The model under review builds one solid part; all positions refer to its coordinate system, in mm. A direction names the side the tool comes from. Coordinates: 2 decimals unless noted, no trailing zeros. Loops run counter-clockwise (first coordinate to the right, second up) from the corner with the lowest first, then second, coordinate; pieces in that order, holes last. Notation, with made-up numbers: (-36, -11) - (20, -11) arc R19 ccw to (20, -7) - close; hole circle Ø2 at (38.5, 74). An arc over 180 degrees is marked (long way). One line per item, written item: value. Start each with the question number.
1. Insertion check: P1, Ø1.5, axis at y = 1.5, z = -10, coming from the +X side; P2, Ø1.5, axis at x = 34, y = 2, coming from the -Z side; P3, Ø1.5, axis at x = 7.5, y = 1, coming from the -Z side. Each pin has a flat end and moves straight along its axis. Give the tip position at first contact, or say it passes through.
2. Mouldability with a two-part tool opening along X and no side actions: class faces 1 (the face through (-52.23, 1.99, -52.13)), 2 (the face through (-1, 3, -15)), 3 (the face through (-13.922, 1.479, -11.116)), 4 (the face through (81.49, 1.52, 38.52)) as +X half, -X half, draft (parallel to the pull), parting line (faces both ways), or undercut.
3. We need section B-B, the plane z = 0. Give the boundary of the cut face in (x, y).
4. We need section D-D, the plane x = -34.5. Count the separate pieces of the cut face and the enclosed holes in it, then the cut area to 3 significant figures.
5. We need section C-C, the plane x = 0. Give the boundary of the cut face in (y, z), then the cut area to 3 significant figures.
6. To check wall thickness, follow line 1 (Z direction, x = -38.5, y = -6.75); line 2 (X direction, y = -3, z = 39.5); line 3 (Z direction, x = -39.1, y = 2.2). State the ranges of each line that lie inside material, in increasing order.
7. For faces 5 (the face through (-52.13, 1.99, 52.23)), 6 (the face through (-18.5, -8, -37.5)), 7 (the face through (-51.465, -3.944, -58.494)), list the 3-axis set-ups (+Z, -Z, +X, -X, +Y, -Y) from which the entire face can be reached by the end or side of a thin tool; tool diameter is ignored.
8. We need section A-A, the plane y = -2.75. Give the boundary of the cut face in (x, z), then the cut area to 3 significant figures.
from build123d import *

# Parameters (mm, degrees)
SKETCH1_W             = 120.2
SKETCH1_H             = 120.2
SKETCH1_W_2           = 110.2
SKETCH1_H_2           = 110.2
BOSS_EXTRUDE1_DEPTH   = 3
SKETCH3_W             = 25
SKETCH3_H             = 25
SKETCH3_R             = 3
SKETCH3_W_2           = 24.35
SKETCH3_H_2           = 24.35
BOSS_EXTRUDE3_DEPTH   = 3
FILLET1_R             = 12
SKETCH4_R             = 26.20371479
SKETCH4_R_2           = 18.5
BOSS_EXTRUDE4_DEPTH   = 3
SKETCH5_R             = 23
SKETCH5_R_2           = 20.5
BOSS_EXTRUDE5_DEPTH   = 8
SKETCH6_R             = 14.298791064
BOSS_EXTRUDE6_DEPTH   = 5.7
CIRPATTERN1_COUNT     = 4
SKETCH7_R             = 21.686675293
CUT_EXTRUDE1_DEPTH    = 5.7
SKETCH8_W             = 5.547879072
SKETCH8_H             = 55.825533157
SKETCH8_W_2           = 52.326060464
SKETCH8_H_2           = 5.547879072
BOSS_EXTRUDE7_DEPTH   = 3
BOSS_EXTRUDE8_DEPTH   = 3
BOSS_EXTRUDE9_DEPTH   = 3
CUT_EXTRUDE2_START    = -9
SKETCH12_R            = 20.5
CUT_EXTRUDE2_DEPTH    = 9
SKETCH14_R            = 1.812502671
CUT_EXTRUDE3_DEPTH    = 9
CIRPATTERN2_OUTLINE_R = 20.5
CIRPATTERN2_DEPTH     = 1


# Read off the part's stored shape, not the designer's step: CirPattern2
with BuildPart() as part:
    # Sketch1 → Boss-Extrude1 (new body)
    with BuildSketch(Plane(origin=(0, 0, 0), x_dir=(1, 0, 0), z_dir=(0, 1, 0))):
        Rectangle(SKETCH1_W, SKETCH1_H)
        Rectangle(SKETCH1_W_2, SKETCH1_H_2, mode=Mode.SUBTRACT)
    extrude(amount=BOSS_EXTRUDE1_DEPTH)

    # Sketch3 → Boss-Extrude3 (add)
    # profile 1 of 4: a face of its own
    with BuildSketch(Plane(origin=(0, 0, 0), x_dir=(-1, 0, 0), z_dir=(0, -1, 0))):
        with Locations((72.6, -47.6)):
            Rectangle(SKETCH3_W, SKETCH3_H)
        with Locations(Location((75.1, -50.1, 0), (0, 0, 90))):
            Circle(SKETCH3_R, mode=Mode.SUBTRACT)
    # profile 2 of 4: a face of its own
    with BuildSketch(Plane(origin=(0, 0, 0), x_dir=(-1, 0, 0), z_dir=(0, -1, 0))):
        with Locations((-72.6, -47.6)):
            Rectangle(SKETCH3_W, SKETCH3_H)
        with Locations(Location((-74.9, -50.1, 0), (0, 0, 90))):
            Circle(SKETCH3_R, mode=Mode.SUBTRACT)
    # profile 3 of 4: a face of its own
    with BuildSketch(Plane(origin=(0, 0, 0), x_dir=(-1, 0, 0), z_dir=(0, -1, 0))):
        with Locations((72.6, 47.6)):
            Rectangle(SKETCH3_W, SKETCH3_H)
        with Locations(Location((75.1, 49.9, 0), (0, 0, 90))):
            Circle(SKETCH3_R, mode=Mode.SUBTRACT)
    # profile 4 of 4: a face of its own
    with BuildSketch(Plane(origin=(0, 0, 0), x_dir=(-1, 0, 0), z_dir=(0, -1, 0))):
        with Locations((-72.275, 47.925)):
            Rectangle(SKETCH3_W_2, SKETCH3_H_2)
        with Locations(Location((-75.260238187, 49.598128293, 0), (0, 0, 90))):
            Circle(SKETCH3_R, mode=Mode.SUBTRACT)
    extrude(amount=-BOSS_EXTRUDE3_DEPTH)

    # Fillet1
    fillet1_edges = [part.edges().sort_by_distance(p)[0] for p in [
        (-60.1, 1.5, 35.1),
        (-85.1, 1.5, 35.1),
        (-85.1, 1.5, 60.1),
        (-60.1, 1.5, -35.1),
        (-85.1, 1.5, -60.1),
        (-85.1, 1.5, -35.1),
        (85.1, 1.5, 60.1),
        (85.1, 1.5, 35.1),
        (60.1, 1.5, 35.1),
        (84.45, 1.5, -60.1),
        (60.1, 1.5, -35.75),
        (84.45, 1.5, -35.75),
    ]]
    fillet(fillet1_edges, radius=FILLET1_R)

    # Sketch4 → Boss-Extrude4 (add)
    with BuildSketch(Plane(origin=(0, 0, 0), x_dir=(-1, 0, 0), z_dir=(0, -1, 0))):
        with Locations((39.1, -39.1)):
            Circle(SKETCH4_R)
        with Locations((39.1, -39.1)):
            Circle(SKETCH4_R_2, mode=Mode.SUBTRACT)
    boss_extrude4 = extrude(amount=-BOSS_EXTRUDE4_DEPTH)

    # Sketch5 → Boss-Extrude5 (add)
    with BuildSketch(Plane(origin=(0, 0, 0), x_dir=(-1, 0, 0), z_dir=(0, -1, 0))):
        with Locations(Location((39.1, -39.1, 0), (0, 0, 270))):
            Circle(SKETCH5_R)
        with Locations(Location((39.1, -39.1, 0), (0, 0, 90))):
            Circle(SKETCH5_R_2, mode=Mode.SUBTRACT)
    boss_extrude5 = extrude(amount=BOSS_EXTRUDE5_DEPTH)

    # CirPattern1: Boss-Extrude4, Boss-Extrude5 ×4 about axis
    cirpattern1_axis = Axis((0, 0, 0), (0, 1, 0))
    add([boss_extrude4.rotate(cirpattern1_axis, i * 360 / CIRPATTERN1_COUNT) for i in range(1, CIRPATTERN1_COUNT)])
    add([boss_extrude5.rotate(cirpattern1_axis, i * 360 / CIRPATTERN1_COUNT) for i in range(1, CIRPATTERN1_COUNT)])

    # Sketch8 → Boss-Extrude7 (add)
    with BuildSketch(Plane(origin=(0, 0, 0), x_dir=(-1, 0, 0), z_dir=(0, -1, 0))):
        with Locations((0, -30.686706115)):
            Rectangle(SKETCH8_W, SKETCH8_H)
        with Locations((-28.936969768, 0)):
            Rectangle(SKETCH8_W_2, SKETCH8_H_2)
        Rectangle(SKETCH8_W, SKETCH8_H_2)
        with Locations((28.936969768, 0)):
            Rectangle(SKETCH8_W_2, SKETCH8_H_2)
        with Locations((0, 30.686706115)):
            Rectangle(SKETCH8_W, SKETCH8_H)
    extrude(amount=-BOSS_EXTRUDE7_DEPTH)

    # Sketch9 → Boss-Extrude8 (add)
    with BuildSketch(Plane(origin=(0, 0, 0), x_dir=(-1, 0, 0), z_dir=(0, -1, 0))):
        Polygon((22.82424649, 20.034817185), (-19.99324685, -22.860669453), (-22.82424649, -20.034817185), (19.99324685, 22.860669453), align=None)
    extrude(amount=-BOSS_EXTRUDE8_DEPTH)

    # Sketch10 → Boss-Extrude9 (add)
    with BuildSketch(Plane(origin=(0, 0, 0), x_dir=(-1, 0, 0), z_dir=(0, -1, 0))):
        Polygon((23.384125812, -20.554528832), (-20.555773995, 23.383031261), (-23.384125812, 20.554528832), (20.555773995, -23.383031261), align=None)
    extrude(amount=-BOSS_EXTRUDE9_DEPTH)

    # Sketch12 → Cut-Extrude2 (cut)
    with BuildSketch(Plane(origin=(0, -8, 0), x_dir=(-1, 0, 0), z_dir=(0, -1, 0)).offset(CUT_EXTRUDE2_START)):
        with Locations(Location((39.1, -39.1, 0), (0, 0, 90))):
            Circle(SKETCH12_R)
    extrude(amount=CUT_EXTRUDE2_DEPTH, mode=Mode.SUBTRACT)

    # Sketch14 → Cut-Extrude3 (cut)
    with BuildSketch(Plane(origin=(0, 0, 0), x_dir=(-1, 0, 0), z_dir=(0, -1, 0))):
        with Locations(Location((0, 0, 0), (0, 0, 90))):
            Circle(SKETCH14_R)
    extrude(amount=-CUT_EXTRUDE3_DEPTH, mode=Mode.SUBTRACT)

    # CirPattern2 outline → CirPattern2 (cut)
    # profile 1 of 3: a face of its own
    with BuildSketch(Plane(origin=(0, 0, 0), x_dir=(1, 0, 0), z_dir=(0, 1, 0))):
        with Locations((39.1, -39.1)):
            Circle(CIRPATTERN2_OUTLINE_R)
        with BuildLine():
            ThreePointArc((55.1, -48.387087811), (52.181475452, -52.181475452), (48.387087811, -55.1))
            Line((48.387087811, -55.1), (29.812912189, -55.1))
            ThreePointArc((29.812912189, -55.1), (26.018524548, -26.018524548), (55.1, -29.812912189))
            Line((55.1, -29.812912189), (55.1, -48.387087811))
        make_face(mode=Mode.SUBTRACT)
    # profile 2 of 3: a face of its own
    with BuildSketch(Plane(origin=(0, 0, 0), x_dir=(1, 0, 0), z_dir=(0, 1, 0))):
        with Locations((39.1, 39.1)):
            Circle(CIRPATTERN2_OUTLINE_R)
        with BuildLine():
            ThreePointArc((55.1, 29.812912189), (26.018524548, 26.018524548), (29.812912189, 55.1))
            Line((29.812912189, 55.1), (48.387087811, 55.1))
            ThreePointArc((48.387087811, 55.1), (52.181475452, 52.181475452), (55.1, 48.387087811))
            Line((55.1, 48.387087811), (55.1, 29.812912189))
        make_face(mode=Mode.SUBTRACT)
    # profile 3 of 3: a face of its own
    with BuildSketch(Plane(origin=(0, 0, 0), x_dir=(1, 0, 0), z_dir=(0, 1, 0))):
        with Locations((-39.1, 39.1)):
            Circle(CIRPATTERN2_OUTLINE_R)
        with BuildLine():
            ThreePointArc((-29.812912189, 55.1), (-26.018524548, 26.018524548), (-55.1, 29.812912189))
            Line((-55.1, 29.812912189), (-55.1, 48.387087811))
            ThreePointArc((-55.1, 48.387087811), (-52.181475452, 52.181475452), (-48.387087811, 55.1))
            Line((-48.387087811, 55.1), (-29.812912189, 55.1))
        make_face(mode=Mode.SUBTRACT)
    extrude(amount=CIRPATTERN2_DEPTH, mode=Mode.SUBTRACT)


with BuildPart() as body_2:
    # Sketch6 → Boss-Extrude6 (new body)
    with BuildSketch(Plane(origin=(0, 0, 0), x_dir=(1, 0, 0), z_dir=(0, 1, 0))):
        with Locations(Location((0, 0, 0), (0, 0, 270))):
            Circle(SKETCH6_R)
    extrude(amount=BOSS_EXTRUDE6_DEPTH)

    # Sketch7 → Cut-Extrude1 (cut)
    with BuildSketch(Plane(origin=(0, 0, 0), x_dir=(-1, 0, 0), z_dir=(0, -1, 0))):
        Circle(SKETCH7_R)
    extrude(amount=-CUT_EXTRUDE1_DEPTH, mode=Mode.SUBTRACT)


solid = part.part
Findings below:
1. P1: x = 60.1
1. P2: z = -64.94
1. P3: z = -60.1
2. face 1: undercut
2. face 2: draft
2. face 3: undercut
2. face 4: +X half
3. outline: (-60.1, 0) - (-1.81, 0) - (-1.81, 3) - (-60.1, 3) - close; (1.81, 0) - (60.1, 0) - (60.1, 3) - (1.81, 3) - close
4. separate pieces: 5
4. enclosed holes: 0
4. area: 192 mm2
5. outline: (0, -60.1) - (3, -60.1) - (3, -1.81) - (0, -1.81) - close; (0, 1.81) - (3, 1.81) - (3, 60.1) - (0, 60.1) - close
5. area: 350 mm2
6. line 1: -62.09 to -59.59, -18.61 to -16.11, 16.11 to 18.61, 59.59 to 62.09
6. line 2: -62.1 to -59.6, -18.6 to -16.1, 16.1 to 18.6, 59.6 to 62.1
6. line 3: -65.3 to -55.1, -20.6 to -12.9, -2.77 to 2.77, 12.9 to 20.6, 55.1 to 65.3
7. face 5: +Y, -Y
7. face 6: +Z, -Z, +X, -X, -Y
7. face 7: -Y
8. outline: circle Ø46 at (-39.1, -39.1); circle Ø46 at (-39.1, 39.1); circle Ø46 at (39.1, -39.1); circle Ø46 at (39.1, 39.1); hole circle Ø41 at (-39.1, -39.1); hole circle Ø41 at (-39.1, 39.1); hole circle Ø41 at (39.1, -39.1); hole circle Ø41 at (39.1, 39.1)
8. area: 1,370 mm2
